For this review, use the dimensioned drawing (mm, ordinates from the lowest corner) and the shaded views. Coordinates: 2 decimals unless noted, no trailing zeros. Loops run counter-clockwise (first coordinate to the right, second up) from the corner with the lowest first, then second, coordinate; pieces in that order, holes last. Notation, with made-up numbers: M 84.25,16.5 L 112.25,16.5 A26 cw 112.25,35.5 Z; hole C 39,10 d1. An arc over 180 degrees is marked long. Use CSV: the item, a comma, the result in double quotes. Start each with the question number.
1. Draft analysis for pull direction Y (two halves, no side actions). For the marked faces 1, 2 and 3, state which applies: +Y half, -Y half, draft (parallel to the pull), parting line (faces both ways), or undercut.
2. Add section B-B, the plane y = 25. Write out the cut boundary in (x, z), then the cut area to 3 significant figures.
3. Add section C-C, the plane z = 2.25. State how many separate pieces and enclosed holes the cut face has, then the cut area to 3 significant figures.
4. Add section D-D, the plane x = 75. Write out the cut boundary in (y, z).
5. Clearance check with a flat-ended pin moving along its axis: P1, Ø10, axis at x = 42, y = 12.5, coming from the -Z side. State where the tip first meets the part, or that it passes through.
6. For L1, parallel to Y at x = 25, z = 5.25; L2, parallel to Y at x = 75, z = 6.75; L3, parallel to X at y = 24.5, z = 5.25, list the stretches that pass through material, from the lowest coordinate up.
7. Add section A-A, the plane x = 25. Write out the cut boundary in (y, z), then the cut area to 3 significant figures.
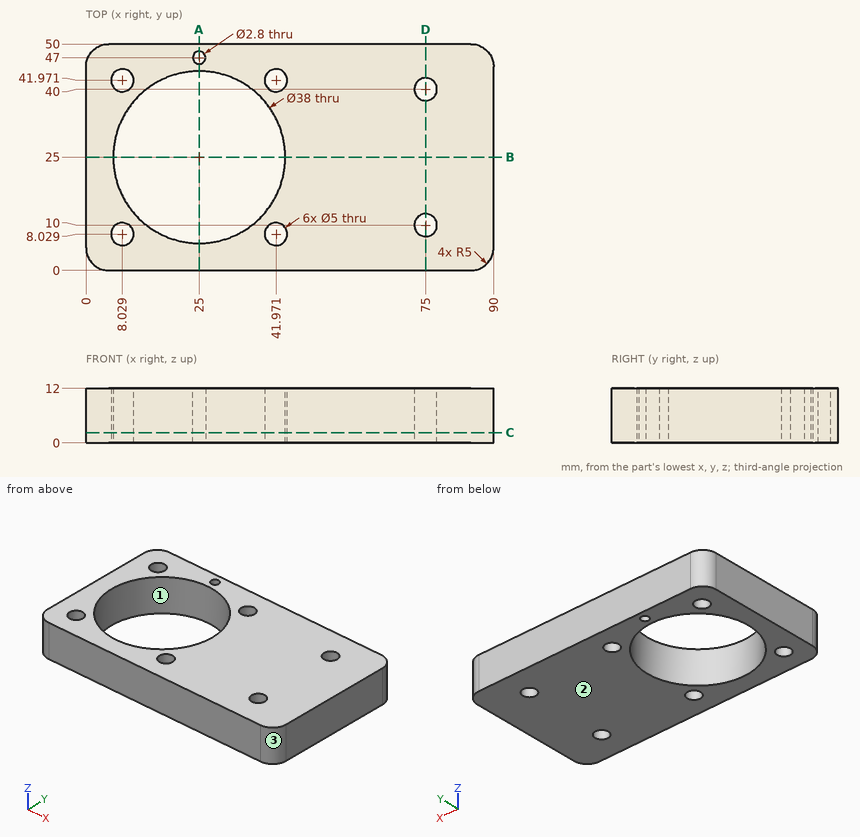
Computed:
1,face 1,"undercut"
1,face 2,"draft"
1,face 3,"-Y half"
2,outline,"M 0,0 L 6,0 L 6,12 L 0,12 Z; M 44,0 L 90,0 L 90,12 L 44,12 Z"
2,area,"624 mm^2"
3,separate pieces,"1"
3,enclosed holes,"8"
3,area,"3,220 mm^2"
4,outline,"M 0,0 L 7.5,0 L 7.5,12 L 0,12 Z; M 12.5,0 L 37.5,0 L 37.5,12 L 12.5,12 Z; M 42.5,0 L 50,0 L 50,12 L 42.5,12 Z"
5,P1,"stops at z = 0"
6,L1,"y = 0 to 6, 44 to 45.6, 48.4 to 50"
6,L2,"y = 0 to 7.5, 12.5 to 37.5, 42.5 to 50"
6,L3,"x = 0 to 6.01, 43.99 to 90"
7,outline,"M 0,0 L 6,0 L 6,12 L 0,12 Z; M 44,0 L 45.6,0 L 45.6,12 L 44,12 Z; M 48.4,0 L 50,0 L 50,12 L 48.4,12 Z"
7,area,"110 mm^2"
